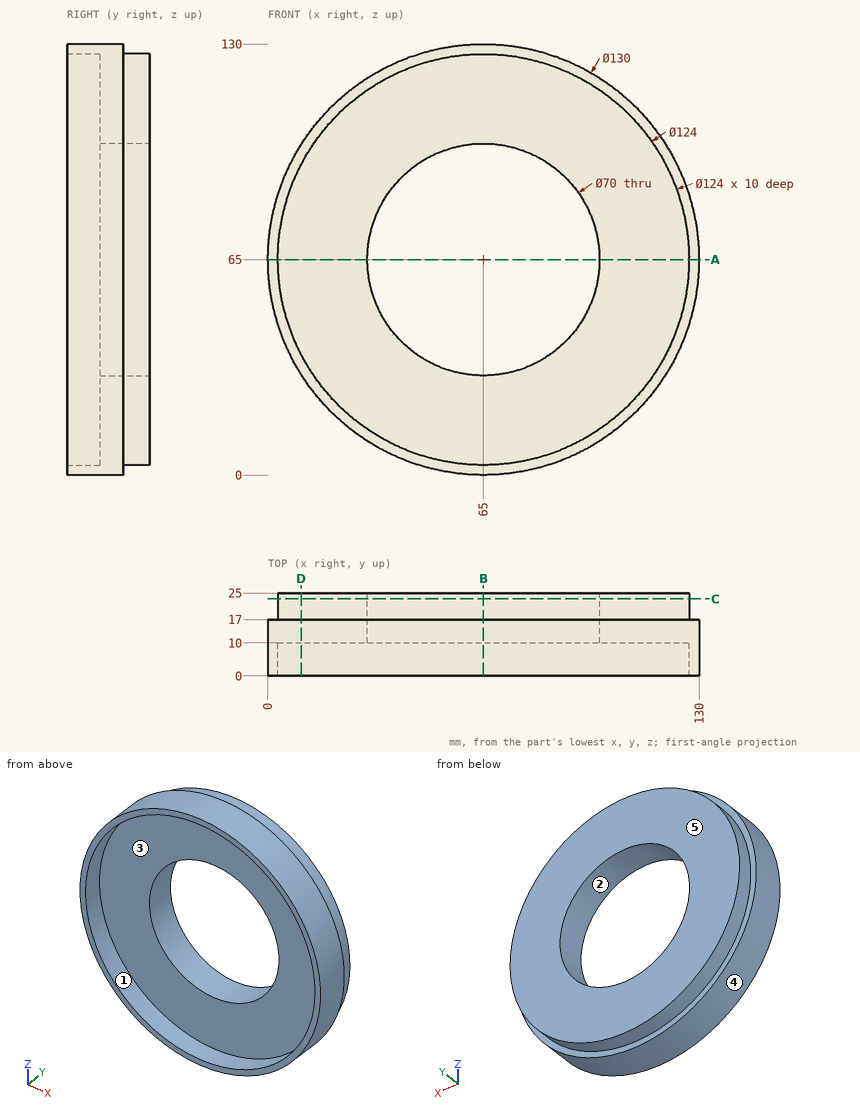
Geometry: see drawing. Coordinates: mm, zero at the bounding-box minimum. A direction names the side the tool comes from. Give positions to 0.01 mm unless a question says otherwise; leave off trailing zeros. Write each loop counter-clockwise with the first axis right and the second up, starting at its lowest first coordinate (ties: lowest second). Pieces come first, ordered by that corner, then holes. Notation, with made-up numbers: (-26, 42) - (23, 42) arc R4 ccw to (23, 47) - close; hole circle Ø3 at (26.25, 45). An arc over 180 degrees is marked (long way). Return JSON: item names as keys, results as strings. Group by question number.
1) Mould query, pull axis Z, two halves, no side actions, for the marked faces 3, 4 and 5. Classes: released by +Z, released by -Z, zero draft, split by the parting line, or undercut.
2) Section A-A on z = 65. Return the cut outline in (x, y).
3) Line query: line 1 (X direction, y = 3.25, z = 65); line 2 (Y direction, x = 115.5, z = 75.5); line 3 (X direction, y = 5, z = 85). Output: solid intervals per line, ascending.
4) First-contact query: P1, Ø3, axis at x = 46, z = 90.5, coming from the +Y side; P2, Ø4, axis at y = 15.5, z = 63, coming from the -X side; P3, Ø3, axis at x = 73, y = 10.5, coming from the +Z side; P4, Ø2, axis at x = 17.5, y = 15.5, coming from the -Z side. Flat tips, straight axial feed; report the tip coordinate or a pass-through.
5) Set-up query: the marked faces 1 and 2. Return all of +Z, -Z, +X, -X, +Y, -Y with unobstructed straight access to the full face (end or side cutting, diameter ignored); none if empty.
6) Section B-B on x = 65. Return the cut outline in (y, z), plus the area to 3 significant figures.
7) Section C-C on y = 23.25. Return the cut outline in (x, z).
8) Section D-D on x = 10. Return the cut outline in (y, z), plus the area to 3 significant figures.
Filled in:
{
 "1": {"face 3": "undercut", "face 4": "split by the parting line", "face 5": "zero draft"},
 "2": {"outline": "(0, 0) - (3, 0) - (3, 10) - (30, 10) - (30, 25) - (3, 25) - (3, 17) - (0, 17) - close; (100, 10) - (127, 10) - (127, 0) - (130, 0) - (130, 17) - (127, 17) - (127, 25) - (100, 25) - close"},
 "3": {"line 1": "x = 0 to 3, 127 to 130", "line 2": "y = 10 to 25", "line 3": "x = 3.15 to 6.31, 123.69 to 126.85"},
 "4": {"P1": "passes through", "P2": "stops at x = 0", "P3": "stops at z = 129.67", "P4": "stops at z = 19.58"},
 "5": {"face 1": "-Y", "face 2": "+Y, -Y"},
 "6": {"outline": "(0, 0) - (17, 0) - (17, 3) - (25, 3) - (25, 30) - (10, 30) - (10, 3) - (0, 3) - close; (0, 127) - (10, 127) - (10, 100) - (25, 100) - (25, 127) - (17, 127) - (17, 130) - (0, 130) - close", "area": "912 mm^2"},
 "7": {"outline": "circle Ø124 at (65, 65); hole circle Ø70 at (65, 65)"},
 "8": {"outline": "(0, 30.36) - (17, 30.36) - (17, 36.38) - (25, 36.38) - (25, 93.62) - (17, 93.62) - (17, 99.64) - (0, 99.64) - (0, 93.62) - (10, 93.62) - (10, 36.38) - (0, 36.38) - close", "area": "1,060 mm^2"}
}
